Build history of the part. All positions in model axes, mm. Face numbers are marked on the shaded views. A direction names the side the tool comes from. Give positions to 0.01 mm unless a question says otherwise; leave off trailing zeros. Order: outer loops, then holes, each group sorted by start corner. A loop starts at its lowest first (then second) coordinate and runs counter-clockwise, first axis right, second up. Notation, with made-up numbers: (22.5, 11) - (79.5, 11) arc R18 ccw to (79.5, 46) - close; hole circle Ø11 at (79.5, 26.25). An arc over 180 degrees is marked (long way). Write each question's results on one line, items separated by ' | '. Start each with the question number.
Autodesk Inventor part; units mm, degrees
ref_plane "YZ Plane" through (0, 0, 0) normal (1, 0, 0) x (0, 1, 0)
ref_plane "XZ Plane" through (0, 0, 0) normal (0, 1, 0) x (-1, 0, 0)
ref_plane "XY Plane" through (0, 0, 0) normal (0, 0, 1) x (1, 0, 0)
sketch "Sketch1" plane through (0, 0, 0) normal (0, 1, 0) x (-1, 0, 0)
  circle A0 centre (0, 11.1484) radius 5.5
  line L0 (0, 11.1484) -> (0, -0.3516)
  circle A1 centre (0, -0.3516) radius 5.5
  circle A2 centre (0, 11.1484) radius 2.5
  circle A3 centre (0, -0.3516) radius 2.5
  line L1 (5.5, 11.1484) -> (5.5, -0.3516)
  line L2 (-5.5, 11.1484) -> (-5.5, -0.3516)
  point P0 (0, 0)
  dimension "d0" = 11
  dimension "d1" = 11.5
  dimension "d2" = 11
  dimension "d3" = 5
  dimension "d4" = 5
extrude "Extrusion1" add sketch "Sketch1" along normal blind 2
sketch "Sketch2" plane through (0, 2, 0) normal (0, 1, 0) x (1, 0, 0)
  circle A0 centre (0, -11.1484) radius 2.5
  line L0 (0, -8.6484) -> (0, -2.1484)
  circle A1 centre (0, 0.3516) radius 2.5
  line L1 (-5.5, 0.3516) -> (-5.5, -11.1484)
  line L2 (5.5, -3.3984) -> (-5.5, -3.3984)
  line L3 (-5.5, -3.3984) -> (-5.5, -7.3984)
  line L4 (-5.5, -7.3984) -> (5.5, -7.3984)
  line L5 (5.5, -7.3984) -> (5.5, -3.3984)
  line L6 (5.5, -3.3984) -> (-5.5, -7.3984) construction
  line L7 (-5.5, -3.3984) -> (5.5, -7.3984) construction
  point P0 (0, 0)
  point P1 (0, -5.3984)
  dimension "d7" = 4
extrude "Extrusion2" add sketch "Sketch2" along normal blind 4 contours L4 L1 L2 L0 | L0 L2 L5 L4
sketch "Sketch3" plane through (0, 6, 0) normal (0, 1, 0) x (1, 0, 0)
  line L0 (5.5, -3.3984) -> (-5.5, -3.3984)
  line L1 (-5.5, -3.3984) -> (-5.5, -7.3984)
  line L2 (-5.5, -7.3984) -> (5.5, -7.3984)
  line L3 (5.5, -7.3984) -> (5.5, -3.3984)
  circle A0 centre (0, -5.3984) radius 1.5
  point P0 (0, 0)
  dimension "d14" = 3
extrude "Extrusion3" cut sketch "Sketch3" against normal blind 16.6375 contours A0
properties part number "bearing plate"
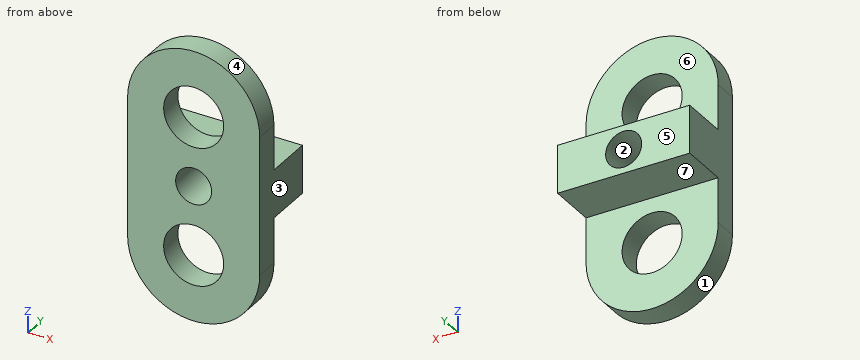
Item 1: Cut at D-D, the plane y = 4.8. List the corners of the cut face in (x, z).
Item 2: Cut at B-B, the plane z = 10. List the corners of the cut face in (x, y), then the cut area to 3 significant figures.
Item 3: Flat gauge pins, fed straight in: pin 1 Ø3 at (x, y) = (1, 4) entering from +Z; pin 2 Ø4.5 at (x, z) = (2.5, -3) entering from +Y. Where does each tip first touch, or does it go through?
Item 4: Which spindle directions (+Z, -Z, +X, -X, +Y, -Y) get a long thin tool onto all of the face, cutting with end or side? Do the marked faces 5, 6 and 7. Say none if no direction does.
Item 5: Two-plate mould, pull along Z, no slides. Class the marked faces 1, 2, 3 and 4: +Z half, -Z half, draft (parallel to the pull), parting line (faces both ways), or undercut.
Item 6: Probe line 1 along Z through (x, y) = (0, 1.35); line 2 along Z through (x, y) = (0, 4.5); line 3 along Y through (x, z) = (2.25, 12.5). List the from-to ranges inside material, lowest first. Write a range as from..to.
Item 7: Cut at A-A, the plane x = 0. List the corners of the cut face in (y, z).
Item 8: Cut at C-C, the plane x = 2. List the corners of the cut face in (y, z), then the cut area to 3 significant figures.
Values found:
1) outline: (-5.5, 3.4) - (5.5, 3.4) - (5.5, 7.4) - (-5.5, 7.4) - close; hole circle Ø3 at (0, 5.4)
2) outline: (-5.5, 0) - (-2.22, 0) - (-2.22, 2) - (-5.5, 2) - close; (2.22, 0) - (5.5, 0) - (5.5, 2) - (2.22, 2) - close | area: 13.1 mm2
3) pin 1: stops at z = 7.4 | pin 2: stops at y = 2
4) face 5: +Z, -Z, +X, -X, +Y | face 6: +Z, +X, -X, +Y | face 7: -Z, +X, -X, +Y
5) face 1: -Z half | face 2: undercut | face 3: draft | face 4: +Z half
6) line 1: z = -5.85..-2.85, 2.15..3.9, 6.9..8.65, 13.65..16.65 | line 2: z = 3.4..3.9, 6.9..7.4 | line 3: y = 0..2
7) outline: (0, -5.85) - (2, -5.85) - (2, -2.85) - (0, -2.85) - close; (0, 2.15) - (2, 2.15) - (2, 3.4) - (6, 3.4) - (6, 3.9) - (0, 3.9) - close; (0, 6.9) - (6, 6.9) - (6, 7.4) - (2, 7.4) - (2, 8.65) - (0, 8.65) - close; (0, 13.65) - (2, 13.65) - (2, 16.65) - (0, 16.65) - close
8) outline: (0, -5.48) - (2, -5.48) - (2, -1.85) - (0, -1.85) - close; (0, 1.15) - (2, 1.15) - (2, 3.4) - (6, 3.4) - (6, 7.4) - (2, 7.4) - (2, 9.65) - (0, 9.65) - close; (0, 12.65) - (2, 12.65) - (2, 16.27) - (0, 16.27) - close | area: 47.5 mm2
